```python
from build123d import *

# Parameters (mm, degrees)
F0_R          = 20
F1_DEPTH      = 110
F1_DEPTH_BACK = 110
F2_W          = 0.8
F2_H          = 13


with BuildPart() as f1:
    # F0 (on Right) → F1 (new body, two sides)
    with BuildSketch(Plane.YZ) as f1_sk:
        Circle(F0_R)
    extrude(amount=F1_DEPTH)
    extrude(f1_sk.sketch, amount=-F1_DEPTH_BACK)

    # F2 (on Front) → F3 (revolve)
    with BuildSketch(Plane.XZ):
        with Locations((-108.6, 23.5)):
            Rectangle(F2_W, F2_H)
        with Locations((-100.6, 23.5)):
            Rectangle(F2_W, F2_H)
        with Locations((-92.6, 23.5)):
            Rectangle(F2_W, F2_H)
        with Locations((-84.6, 23.5)):
            Rectangle(F2_W, F2_H)
        with Locations((-76.6, 23.5)):
            Rectangle(F2_W, F2_H)
        with Locations((-68.6, 23.5)):
            Rectangle(F2_W, F2_H)
        with Locations((-60.6, 23.5)):
            Rectangle(F2_W, F2_H)
        with Locations((-52.6, 23.5)):
            Rectangle(F2_W, F2_H)
        with Locations((-44.6, 23.5)):
            Rectangle(F2_W, F2_H)
        with Locations((-36.6, 23.5)):
            Rectangle(F2_W, F2_H)
        with Locations((-28.6, 23.5)):
            Rectangle(F2_W, F2_H)
        with Locations((-20.6, 23.5)):
            Rectangle(F2_W, F2_H)
        with Locations((-12.6, 23.5)):
            Rectangle(F2_W, F2_H)
        with Locations((-4.6, 23.5)):
            Rectangle(F2_W, F2_H)
        with Locations((3.4, 23.5)):
            Rectangle(F2_W, F2_H)
        with Locations((11.4, 23.5)):
            Rectangle(F2_W, F2_H)
        with Locations((19.4, 23.5)):
            Rectangle(F2_W, F2_H)
        with Locations((27.4, 23.5)):
            Rectangle(F2_W, F2_H)
        with Locations((35.4, 23.5)):
            Rectangle(F2_W, F2_H)
        with Locations((43.4, 23.5)):
            Rectangle(F2_W, F2_H)
        with Locations((51.4, 23.5)):
            Rectangle(F2_W, F2_H)
        with Locations((59.4, 23.5)):
            Rectangle(F2_W, F2_H)
        with Locations((67.4, 23.5)):
            Rectangle(F2_W, F2_H)
        with Locations((75.4, 23.5)):
            Rectangle(F2_W, F2_H)
        with Locations((83.4, 23.5)):
            Rectangle(F2_W, F2_H)
        with Locations((91.4, 23.5)):
            Rectangle(F2_W, F2_H)
        with Locations((99.4, 23.5)):
            Rectangle(F2_W, F2_H)
        with Locations((107.4, 23.5)):
            Rectangle(F2_W, F2_H)
    revolve(axis=Axis((0, 0, 0), (-1, 0, 0)))


solid = f1.part
```
The listing builds one solid part. Answer for the finished solid, in the listing's coordinates (mm). A direction names the side the tool comes from. Round coordinates to 2 decimals unless told otherwise and drop trailing zeros. Loops run counter-clockwise (first coordinate to the right, second up) from the corner with the lowest first, then second, coordinate; pieces in that order, holes last.
1) Consider line 1 (Z direction, x = -75, y = -2.5); line 2 (Z direction, x = -63, y = -9); line 3 (Y direction, x = -66.5, z = -13.5). Determine where each line is inside the solid, lowest interval first.
Outcome:
line 1: z = -19.84 to 19.84
line 2: z = -17.86 to 17.86
line 3: y = -14.76 to 14.76
2) For a pull along X with two mould halves and no side action, classify faces 1 (the face through (-110, 0, 0)), 2 (the face through (-76.59, 1.32, -29.97)), 3 (the face through (107.8, -20, -6)), 4 (the face through (19.8, -20, -6)) as released by +X, released by -X, zero draft, split by the parting line, or undercut.
Outcome:
face 1: released by -X
face 2: zero draft
face 3: released by +X
face 4: undercut
3) Given P1, Ø12, axis at x = -50.5, z = 16, coming from the +Y side; P2, Ø8, axis at x = 72.5, z = 12, coming from the +Y side; P3, Ø12, axis at x = 53.5, y = 13.5, coming from the -Z side, each flat-ended and moving along its own axis, determine where each tip first touches the part or whether it passes through.
Outcome:
P1: stops at y = 28.2
P2: stops at y = 28.66
P3: stops at z = -28.98
4) For faces 5 (the face through (99.41, 1.32, -29.97)), 6 (the face through (87.45, -4.336, -19.524)), determine the directions among +Z, -Z, +X, -X, +Y, -Y from which every point of the face is accessible in a straight line to the end or side of a thin tool.
Outcome:
face 5: +X, -X
face 6: none
5) A cutting plane is placed at A-A on x = 55. Determine the outline of the cut face in (y, z).
Outcome:
outline: circle Ø40 at (0, 0)
